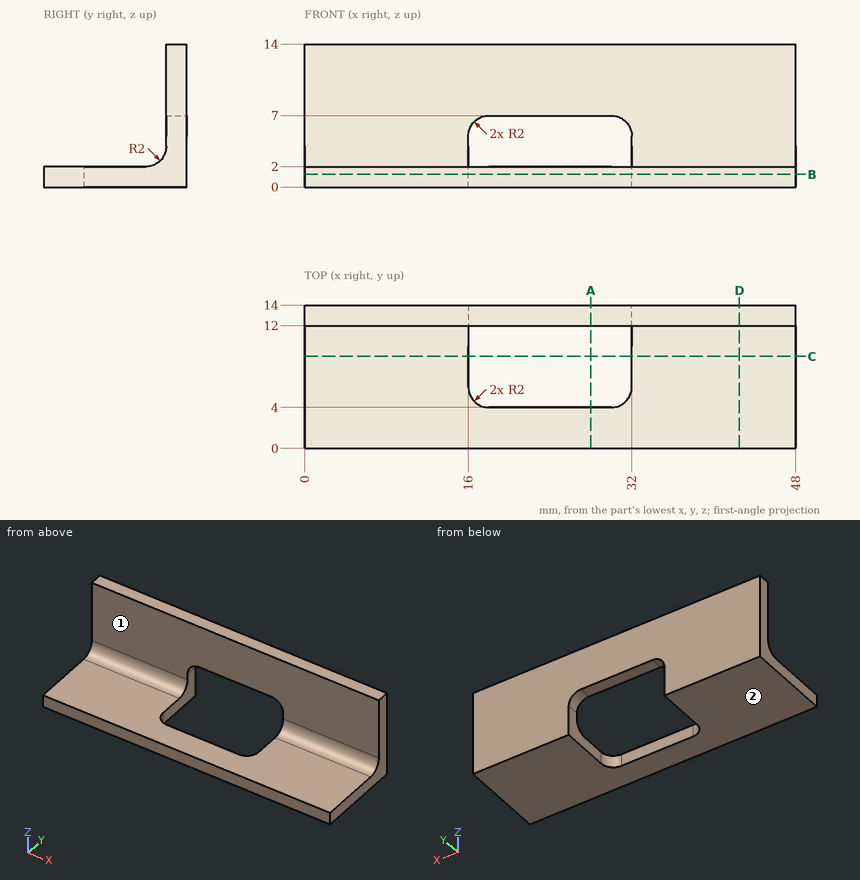
Study the drawing (mm; zero at the part's minimum x, y, z) and answer. A direction names the side the tool comes from. Round coordinates to 2 decimals unless told otherwise and drop trailing zeros. Write each loop counter-clockwise with the first axis right and the second up, starting at its lowest first coordinate (ties: lowest second). Pieces come first, ordered by that corner, then holes. Notation, with made-up numbers: (-22.75, 62.25) - (18.25, 62.25) arc R17 cw to (18.25, 91.25) - close; hole circle Ø2 at (49, 20.5). An arc over 180 degrees is marked (long way). Use a Markdown table: item, result. Add a question column.
1. Flat-ended cylindrical pins translate along their axes: P1, Ø6, axis at y = 11, z = 8, coming from the +X side; P2, Ø8, axis at x = 14, z = 10.5, coming from the -Y side; P3, Ø1.6, axis at x = 26.5, z = 1.5, coming from the +Y side; P4, Ø1.5, axis at x = 19.5, z = 3.5, coming from the +Y side (1 decimal). Find the tip coordinate at first contact, or state that the pin passes through.
2. The part is cut by section B-B (z = 1.25). Write down the section's boundary in (x, y), and give its area (3 significant figures).
3. The part is cut by section A-A (x = 28). Write down the section's boundary in (y, z).
4. The part is cut by section C-C (y = 9). Write down the section's boundary in (x, z).
5. The part is cut by section D-D (x = 42.5). Write down the section's boundary in (y, z), and give its area (3 significant figures).
6. A tool of negligible diameter and unlimited length cuts with its end or side. For the marked faces 1 and 2, from which of +Z, -Z, +X, -X, +Y, -Y can it reach the whole face along a straight path? Write none if from no direction.
7. Consider line 1 (Y direction, x = 3.5, z = 5); line 2 (Z direction, x = 45, y = 7); line 3 (Z direction, x = 6, y = 10.5). Determine where each line is inside the solid, lowest interval first.
Reported:
| question | item | result |
|---|---|---|
| 1 | P1 | x = 48 |
| 1 | P2 | y = 12 |
| 1 | P3 | y = 4 |
| 1 | P4 | through |
| 2 | outline | (0, 0) - (48, 0) - (48, 14) - (32, 14) - (32, 6) arc R2 cw to (30, 4) - (18, 4) arc R2 cw to (16, 6) - (16, 14) - (0, 14) - close |
| 2 | area | 514 mm^2 |
| 3 | outline | (0, 0) - (4, 0) - (4, 2) - (0, 2) - close; (12, 7) - (14, 7) - (14, 14) - (12, 14) - close |
| 4 | outline | (0, 0) - (16, 0) - (16, 2) - (0, 2) - close; (32, 0) - (48, 0) - (48, 2) - (32, 2) - close |
| 5 | outline | (0, 0) - (14, 0) - (14, 14) - (12, 14) - (12, 4) arc R2 cw to (10, 2) - (0, 2) - close |
| 5 | area | 52.9 mm^2 |
| 6 | face 1 | +Z, +X, -X, -Y |
| 6 | face 2 | -Z, +X, -X, +Y, -Y |
| 7 | line 1 | 12 to 14 |
| 7 | line 2 | 0 to 2 |
| 7 | line 3 | 0 to 2.06 |
